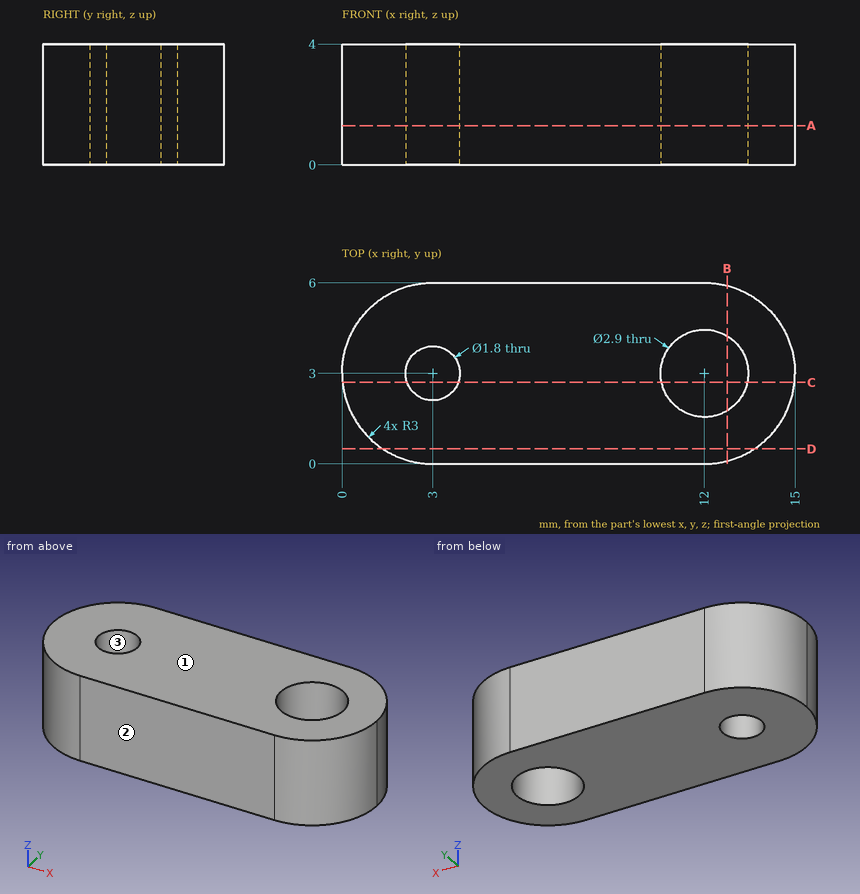
Geometry: see drawing. Coordinates: mm, zero at the bounding-box minimum. Round coordinates to 2 decimals unless told otherwise and drop trailing zeros. Loops run counter-clockwise (first coordinate to the right, second up) from the corner with the lowest first, then second, coordinate; pieces in that order, holes last. Notation, with made-up numbers: M 56,-10.5 L 68,-10.5 A26 cw 68,14.5 Z; hole C 32.25,-38.75 d10. An arc over 180 degrees is marked long. Use a Markdown table: item, result. Add a question column.
1. Cut plane C-C, the plane y = 2.7. Output: boundary loops of the cut face in (x, z) (1 decimal).
2. Cut plane D-D, the plane y = 0.5. Output: boundary loops of the cut face in (x, z).
3. Cut plane A-A, the plane z = 1.3. State how many separate pieces and enclosed holes the cut face has, and give its area (3 significant figures).
4. Contact query for flat-ended pins moving along their axis: pin 1 (1.5 mm diameter, centred on y = 4.5, z = 2, fed in from -X); pin 2 (2.5 mm diameter, centred on x = 3, y = 3, fed in from -Z). Output: stop coordinate, or through.
5. Cut plane B-B, the plane x = 12.75. Output: boundary loops of the cut face in (y, z).
6. Ray query, line 1 along X through (y, z) = (3, 2); line 2 along Y through (x, z) = (12, 1.9); line 3 along X through (y, z) = (3.5, 3.35). Return the intervals inside material, ascending. Write a range as [from, to].
7. Pull-direction query (Y, two-part tool) for the marked faces 1, 2 and 3; classes: +Y half, -Y half, draft (parallel to the pull), parting line (faces both ways), or undercut.
Solution:
| question | item | result |
|---|---|---|
| 1 | outline | M 0,0 L 2.2,0 L 2.2,4 L 0,4 Z; M 3.8,0 L 10.6,0 L 10.6,4 L 3.8,4 Z; M 13.4,0 L 15,0 L 15,4 L 13.4,4 Z |
| 2 | outline | M 1.34,0 L 13.66,0 L 13.66,4 L 1.34,4 Z |
| 3 | separate pieces | 1 |
| 3 | enclosed holes | 2 |
| 3 | area | 73.1 mm2 |
| 4 | pin 1 | stops at x = 0.1 |
| 4 | pin 2 | stops at z = 0 |
| 5 | outline | M 0.1,0 L 1.76,0 L 1.76,4 L 0.1,4 Z; M 4.24,0 L 5.9,0 L 5.9,4 L 4.24,4 Z |
| 6 | line 1 | x = [0, 2.1], [3.9, 10.55], [13.45, 15] |
| 6 | line 2 | y = [0, 1.55], [4.45, 6] |
| 6 | line 3 | x = [0.04, 2.25], [3.75, 10.64], [13.36, 14.96] |
| 7 | face 1 | draft |
| 7 | face 2 | -Y half |
| 7 | face 3 | undercut |
